Part print with two shaded views. Sizes in mm from the minimum x, y, z corner. A direction names the side the tool comes from. Give positions to 0.01 mm unless a question says otherwise; leave off trailing zeros. Write each loop counter-clockwise with the first axis right and the second up, starting at its lowest first coordinate (ties: lowest second). Pieces come first, ordered by that corner, then holes. Notation, with made-up numbers: (86.25, 68.5) - (97.25, 68.5) arc R15 cw to (97.25, 97.5) - close; hole circle Ø7 at (79.5, 0.5). An arc over 180 degrees is marked (long way). Answer as a JSON object with one key per item and string values.
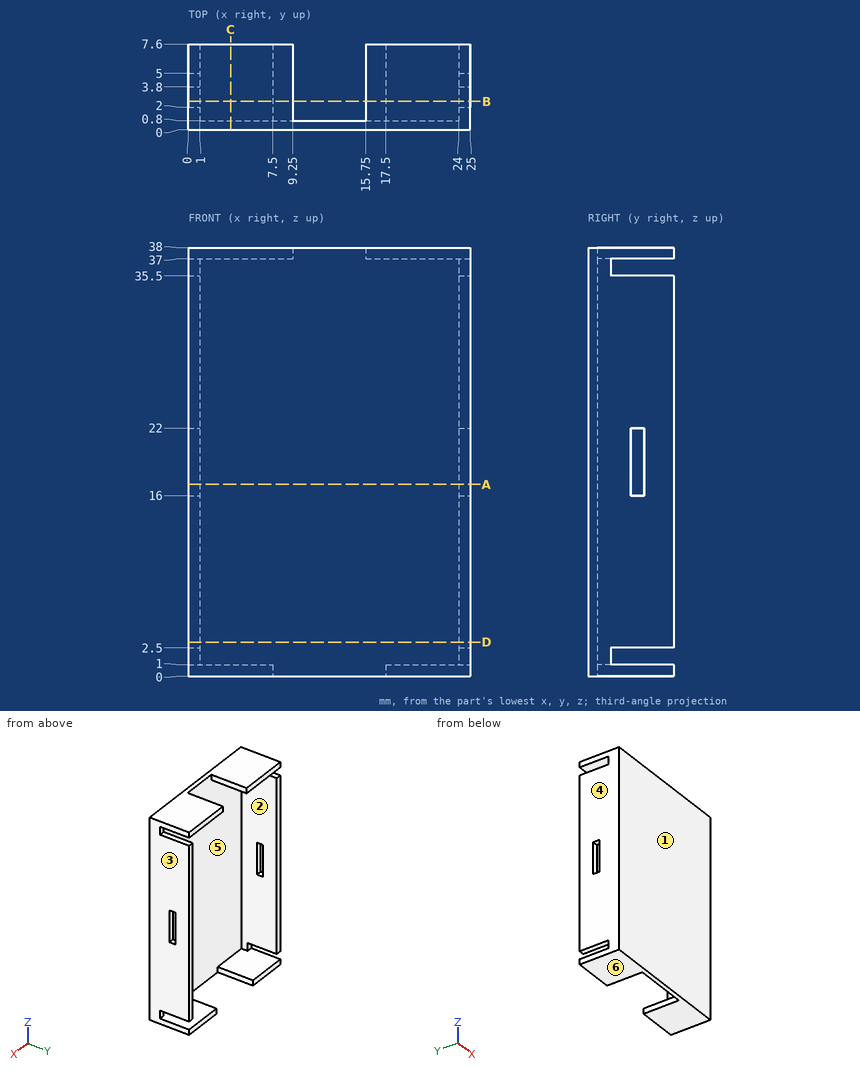
(1) 3-axis set-ups, long thin cutter, end or side, ignore diameter. For the marked faces 1 and 2: which of +Z, -Z, +X, -X, +Y, -Y reach the whole face in a straight line?
Answer key:
{"face 1": "+Z, -Z, +X, -X, -Y", "face 2": "+Y"}
(2) Saw through at D-D, the plane z = 3. Give the cut face in (x, y), and give its area (3 significant figures).
Answer key:
{"outline": "(0, 0) - (25, 0) - (25, 7.6) - (24, 7.6) - (24, 0.8) - (1, 0.8) - (1, 7.6) - (0, 7.6) - close", "area": "33.6 mm²"}
(3) Saw through at B-B, the plane y = 2.5. Give the cut face in (x, z), and give its area (3 significant figures).
Answer key:
{"outline": "(0, 0) - (7.5, 0) - (7.5, 1) - (0, 1) - close; (0, 2.5) - (1, 2.5) - (1, 35.5) - (0, 35.5) - close; (0, 37) - (9.25, 37) - (9.25, 38) - (0, 38) - close; (15.75, 37) - (25, 37) - (25, 38) - (15.75, 38) - close; (17.5, 0) - (25, 0) - (25, 1) - (17.5, 1) - close; (24, 2.5) - (25, 2.5) - (25, 35.5) - (24, 35.5) - close", "area": "99.5 mm²"}
(4) Saw through at A-A, the plane z = 17. Give the cut face in (x, y), and give its area (3 significant figures).
Answer key:
{"outline": "(0, 0) - (25, 0) - (25, 3.8) - (24, 3.8) - (24, 0.8) - (1, 0.8) - (1, 3.8) - (0, 3.8) - close; (0, 5) - (1, 5) - (1, 7.6) - (0, 7.6) - close; (24, 5) - (25, 5) - (25, 7.6) - (24, 7.6) - close", "area": "31.2 mm²"}
(5) Flat gauge pins, fed straight in: P1, Ø0.8, axis at x = 24.5, z = 2, coming from the +Y side; P2, Ø3, axis at x = 6, z = 23, coming from the +Y side; P3, Ø1, axis at x = 16, y = 5.5, coming from the -Z side. Where does each tip first touch, or does it go through?
Answer key:
{"P1": "stops at y = 2", "P2": "stops at y = 0.8", "P3": "stops at z = 37"}
(6) Saw through at C-C, the plane x = 3.75. Give the cut face in (y, z), and give its area (3 significant figures).
Answer key:
{"outline": "(0, 0) - (7.6, 0) - (7.6, 1) - (0.8, 1) - (0.8, 37) - (7.6, 37) - (7.6, 38) - (0, 38) - close", "area": "44.0 mm²"}
(7) Pull direction X, two halves, no side cores. Call the marked faces 3, 4, 5 and 6: pulls with the +X half, pulls with the -X half, needs draft (parallel to the pull), parting line crosses it, or undercut.
Answer key:
{"face 3": "pulls with the +X half", "face 4": "pulls with the -X half", "face 5": "undercut", "face 6": "needs draft"}
(8) Probe L1, parallel to X at y = 6.5, z = 26; L2, parallel to Z at x = 22.75, y = 3.75; L3, parallel to Y at x = 12.5, z = 19.5. List the from-to ranges inside material, lowest first. Write a range as [from, to].
Answer key:
{"L1": "x = [0, 1], [24, 25]", "L2": "z = [0, 1], [37, 38]", "L3": "y = [0, 0.8]"}
